Can you work these out from the model? Positions are in its coordinate system, mm. A direction names the side the tool comes from. Coordinates: 2 decimals unless noted, no trailing zeros. Loops run counter-clockwise (first coordinate to the right, second up) from the corner with the lowest first, then second, coordinate; pieces in that order, holes last. Notation, with made-up numbers: (-30, 29.25) -> (6, 29.25) arc R9 ccw to (6, 34.25) -> close; hole circle Ø8 at (57, -26.5). An arc over 180 degrees is marked (long way). Use one line per item in the form item = value. Start each with the question number.
(1) On a 3-axis mill with a long thin cutter (end or side, diameter ignored), from which of +Z, -Z, +X, -X, +Y, -Y can I reach the whole of each face in a straight line? I mean faces 5 (the cylindrical face through (59.035, -2.958, -12.59)), 6 (the cylindrical face through (18.502, -2.958, 56.946)), 7 (the cylindrical face through (40.444, -2.958, -45.157)). Say none if no direction works.
(2) Imagine slicing it at D-D (y = -3.1). List the corners of the cut face in (x, z) for me, plus the area to 3 significant figures.
(3) Imagine slicing it at A-A (x = 56.5). List the corners of the cut face in (y, z) for me.
(4) Imagine slicing it at C-C (x = 102). List the corners of the cut face in (y, z) for me.
(5) I'm going to push flat-ended pins straight in: pin 1 (3 mm diameter, centred on x = 117, y = -4.5, fed in from +Z) (3 decimals); pin 2 (13 mm diameter, centred on x = 0, z = 0, fed in from -Y). Where does each tip first touch, or does it pass through?
(6) Imagine slicing it at B-B (z = 0). List the corners of the cut face in (x, y) for me.
(7) Thinking about a two-plate mould opening in Z: for faces 1 (the cylindrical face through (-137.65, -2.96, 81.53)), 2 (the cylindrical face through (-91.477, -2.958, 87.194)), 3 (the flat face through (-2, -6, -23)), 4 (the cylindrical face through (-18.47, -2.96, 56.95)), which applies, released by +Z, released by -Z, zero draft, split by the parting line, or undercut?
(8) I need wall thicknesses on line 1 (Z direction, x = 0, y = -3.2); line 2 (X direction, y = -5.35, z = 65.5); line 3 (X direction, y = -2.6, z = 59). Which ranges of each line are inside material? Lowest first, please. Write a range as [from, to].
```python
from build123d import *

# Parameters (mm, degrees)
F0_R        = 37.5
F0_R_2      = 11
F1_DEPTH    = 6
F2_T1_DEPTH = 6


# Not quite as in the source:
# - a fillet or chamfer that OpenCascade refuses, or shapes differently, is made with other operations: its cross-section is extruded or revolved along the edge and cut away or added


with BuildPart() as f1:
    # F0 (on Front) → F1 (new body)
    with BuildSketch(Plane.XZ):
        with BuildLine():
            ThreePointArc((57.8643034804, -2.6875543668), (117.2345315762, -1.6261715812), (146.617452556, 49.9741624513))
            ThreePointArc((146.617452556, 49.9741624513), (87.0017930869, 109.9729314583), (26.6223764775, 50.7428277423))
            ThreePointArc((26.6223764775, 50.7428277423), (34.8220541109, 19.6882465841), (57.8643034804, -2.6875543668))
        make_face()
        with Locations((86.617452556, 49.9741624513)):
            Circle(F0_R, mode=Mode.SUBTRACT)
        with BuildLine():
            ThreePointArc((-26.5950813994, 50.0129171058), (-26.5961913872, 50.3778791758), (-26.5995213098, 50.7428277423))
            ThreePointArc((-26.5995213098, 50.7428277423), (-138.5810142586, 79.97060034), (-57.1442597977, -2.261829254))
            ThreePointArc((-57.1442597977, -2.261829254), (-34.7923339042, 19.7395731883), (-26.5950813994, 50.0129171058))
        make_face()
        with Locations((-86.5950813994, 50.0129171058)):
            Circle(F0_R, mode=Mode.SUBTRACT)
        with BuildLine():
            ThreePointArc((57.8643034804, -2.6875543668), (34.8220541109, 19.6882465841), (26.6223764775, 50.7428277423))
            Line((26.6223764775, 50.7428277423), (-26.5995213098, 50.7428277423))
            ThreePointArc((-26.5995213098, 50.7428277423), (-26.5961913872, 50.3778791758), (-26.5950813994, 50.0129171058))
            ThreePointArc((-26.5950813994, 50.0129171058), (-34.7923339042, 19.7395731883), (-57.1442597977, -2.261829254))
            Line((-57.1442597977, -2.261829254), (-30.1904821111, -48.1489171772))
            ThreePointArc((-30.1904821111, -48.1489171772), (0.418102689, -40.0014567665), (30.9101684744, -48.5746999534))
            Line((30.9101684744, -48.5746999534), (57.8643034804, -2.6875543668))
        make_face()
        Circle(F0_R_2, mode=Mode.SUBTRACT)
        with BuildLine():
            ThreePointArc((60, -100), (52.2236062929, -70.4585893064), (30.9101684744, -48.5746999534))
            ThreePointArc((30.9101684744, -48.5746999534), (0.418102689, -40.0014567665), (-30.1904821111, -48.1489171772))
            ThreePointArc((-30.1904821111, -48.1489171772), (-29.9046072816, -152.0164826121), (60, -100))
        make_face()
        with Locations((0, -100)):
            Circle(F0_R, mode=Mode.SUBTRACT)
    extrude(amount=F1_DEPTH)

    # F2: fillet of radius 35 on 6 edges, made by hand

    # F2_s2 → F2_t1 (join)
    with BuildSketch(Plane.XZ):
        with BuildLine():
            ThreePointArc((-44.5789786986, -23.6534191556), (-39.8361716067, -43.7215717477), (-47.2154351555, -62.9769979192))
            ThreePointArc((-47.2154351555, -62.9769979192), (-39.40668727, -54.7549671411), (-30.1904821111, -48.1489171772))
            Line((-30.1904821111, -48.1489171772), (-44.5789786986, -23.6534191556))
        make_face()
        with BuildLine():
            ThreePointArc((-1.3916525599, 50.7428277423), (18.1502571968, 56.7064064225), (31.0327545881, 72.5648984246))
            ThreePointArc((31.0327545881, 72.5648984246), (27.8065544641, 61.8602158597), (26.6223764775, 50.7428277423))
            Line((26.6223764775, 50.7428277423), (-1.3916525599, 50.7428277423))
        make_face()
        with BuildLine():
            ThreePointArc((1.4297644449, 50.7428277423), (-18.1185373349, 56.7107093642), (-31.0004419188, 72.5791764552))
            ThreePointArc((-31.0004419188, 72.5791764552), (-27.7777362498, 61.8670265011), (-26.5995213098, 50.7428277423))
            Line((-26.5995213098, 50.7428277423), (1.4297644449, 50.7428277423))
        make_face()
        with BuildLine():
            ThreePointArc((43.89611258, -26.4672233966), (58.7364313951, -12.7341703185), (78.6957856647, -9.500598529))
            ThreePointArc((78.6957856647, -9.500598529), (67.9663152116, -7.0533315824), (57.8643034804, -2.6875543668))
            Line((57.8643034804, -2.6875543668), (43.89611258, -26.4672233966))
        make_face()
        with BuildLine():
            ThreePointArc((47.5642084271, -63.4261558392), (40.3776870322, -44.2671300594), (45.1312959448, -24.3644277078))
            Line((45.1312959448, -24.3644277078), (30.9101684744, -48.5746999534))
            ThreePointArc((30.9101684744, -48.5746999534), (39.9336749248, -55.2194059106), (47.5642084271, -63.4261558392))
        make_face()
        with BuildLine():
            ThreePointArc((-78.1330690057, -9.3873720033), (-58.0015888855, -12.5081469238), (-43.0181014785, -26.3107131005))
            Line((-43.0181014785, -26.3107131005), (-57.1442597977, -2.261829254))
            ThreePointArc((-57.1442597977, -2.261829254), (-67.3067666659, -6.8022297719), (-78.1330690057, -9.3873720033))
        make_face()
    extrude(amount=F2_T1_DEPTH)


solid = f1.part
```
Worked out:
q1.face_5 = +Y, -Y
q1.face_6 = +Z, +Y, -Y
q1.face_7 = +X, +Y, -Y
q2.outline = (-78.13, -9.39) arc R35 cw to (-43.83, -25) arc R35 cw to (-47.22, -62.98) arc R60 ccw (long way) to (47.56, -63.43) arc R35 cw to (44.53, -25.43) arc R35 cw to (78.7, -9.5) arc R60 ccw (long way) to (31.03, 72.56) arc R35 cw to (0.02, 50.77) arc R35 cw to (-31, 72.58) arc R60 ccw (long way) to start; hole circle Ø75 at (-86.6, 50.01); hole circle Ø75 at (0, -100); hole circle Ø22 at (0, 0); hole circle Ø75 at (86.62, 49.97)
q2.area = 28,600 mm2
q3.outline = (-6, -120.19) -> (0, -120.19) -> (0, -79.81) -> (-6, -79.81) -> close; (-6, -13.93) -> (0, -13.93) -> (0, 27.63) -> (-6, 27.63) -> close; (-6, 72.32) -> (0, 72.32) -> (0, 101.87) -> (-6, 101.87) -> close
q4.outline = (-6, -8.02) -> (0, -8.02) -> (0, 15.77) -> (-6, 15.77) -> close; (-6, 84.17) -> (0, 84.17) -> (0, 107.97) -> (-6, 107.97) -> close
q5.pin_1 = 102.565
q5.pin_2 = through
q6.outline = (-119.74, -6) -> (-11, -6) -> (-11, 0) -> (-119.74, 0) -> close; (11, -6) -> (119.82, -6) -> (119.82, 0) -> (11, 0) -> close
q7.face_1 = split by the parting line
q7.face_2 = undercut
q7.face_3 = zero draft
q7.face_4 = released by +Z
q8.line_1 = [-160, -137.5], [-62.5, -11], [11, 50.77]
q8.line_2 = [-144.56, -120.75], [-52.44, -27.12], [27.16, 52.48], [120.75, 144.57]
q8.line_3 = [-145.92, -123], [-50.19, -21.15], [21.19, 50.22], [123.02, 145.93]
